The listing builds one solid part. Answer for the finished solid, in the listing's coordinates (mm). A direction names the side the tool comes from. Coordinates: 2 decimals unless noted, no trailing zeros. Write each loop counter-clockwise with the first axis right and the second up, starting at its lowest first coordinate (ties: lowest second). Pieces come first, ordered by that corner, then holes. Notation, with made-up numbers: M 59.25,85 L 112.25,85 A8 cw 112.25,94 Z; hole C 65.5,-29.5 d4. An arc over 180 degrees is marked long. Answer as CSV lines item,"result".
```python
from build123d import *

# Parameters (mm, degrees)
F0_W     = 31.75
F0_H     = 31.75
F1_DEPTH = 1.905
F2_R     = 14.478
F3_DEPTH = 0.889
F5_D     = 1.5875
F6_R     = 1.5875
F7_DEPTH = 3.811
F8_R     = 3.175
F8_R_2   = 1.5875
F9_DEPTH = 2.54


with BuildPart() as f1:
    # F0 (on Front) → F1 (new body, symmetric)
    with BuildSketch(Plane.XZ):
        Rectangle(F0_W, F0_H)
    extrude(amount=F1_DEPTH, both=True)

    # F2 (on face) → F3 (cut)
    with BuildSketch(Plane(origin=(0, 1.905, 0), x_dir=(-1, 0, 0), z_dir=(0, 1, 0))):
        Circle(F2_R)
    extrude(amount=-F3_DEPTH, mode=Mode.SUBTRACT)

    # F5 (through all)
    with Locations(Plane.XZ.offset(1.905)):
        with Locations((-13.335, 13.335), (13.335, 13.335), (13.335, -13.335), (-13.335, -13.335)):
            Hole(F5_D / 2)

    # F6 (on face) → F7 (cut, through all)
    with BuildSketch(Plane.XZ.offset(1.905)):
        Circle(F6_R)
    extrude(amount=-F7_DEPTH, mode=Mode.SUBTRACT)

    # F8 (on face) → F9 (join)
    with BuildSketch(Plane.XZ.offset(1.905)):
        Circle(F8_R)
        Circle(F8_R_2, mode=Mode.SUBTRACT)
    extrude(amount=F9_DEPTH)


solid = f1.part
```
Q1. Find section D-D (x = 6.5). Give the vertices of the cut face in (y, z) (3 decimals), and give its area (3 significant figures).
Output:
outline,"M -1.905,-15.875 L 1.905,-15.875 L 1.905,-12.937 L 1.016,-12.937 L 1.016,12.937 L 1.905,12.937 L 1.905,15.875 L -1.905,15.875 Z"
area,"98.0 mm2"
Q2. Find section B-B (z = 0). Give the vertices of the cut face in (x, y) (1 decimal).
Output:
outline,"M -15.9,-1.9 L -3.2,-1.9 L -3.2,-4.4 L -1.6,-4.4 L -1.6,1 L -14.5,1 L -14.5,1.9 L -15.9,1.9 Z; M 1.6,-4.4 L 3.2,-4.4 L 3.2,-1.9 L 15.9,-1.9 L 15.9,1.9 L 14.5,1.9 L 14.5,1 L 1.6,1 Z"
Q3. Find section A-A (x = 0). Give the vertices of the cut face in (y, z) (1 decimal).
Output:
outline,"M -4.4,-3.2 L -1.9,-3.2 L -1.9,-15.9 L 1.9,-15.9 L 1.9,-14.5 L 1,-14.5 L 1,-1.6 L -4.4,-1.6 Z; M -4.4,1.6 L 1,1.6 L 1,14.5 L 1.9,14.5 L 1.9,15.9 L -1.9,15.9 L -1.9,3.2 L -4.4,3.2 Z"
Q4. Straight lines are drawn through the part: line 1 (Z direction, x = 0, y = 1.45) (3 decimals); line 2 (Z direction, x = 13, y = 1.5) (3 decimals); line 3 (Y direction, x = -12, z = 15) (3 decimals). For each, find the intervals that lie inside material, in ascending order.
Output:
line 1,"-15.875 to -14.478, 14.478 to 15.875"
line 2,"-15.875 to -14.055, -12.615 to -6.373, 6.373 to 12.615, 14.055 to 15.875"
line 3,"-1.905 to 1.905"
Q5. A flat-ended cylindrical pin translates along its axis: pin 1 Ø4 at (x, z) = (10.5, 5.5) entering from -Y (3 decimals). Find the tip coordinate at first contact, or state that the pin passes through.
Output:
pin 1,"y = -1.905"
Q6. For faces 4 (the cylindrical face through (1.885, 1.467, 14.355)), 5 (the cylindrical face through (13.965, 0.027, -13.818)), determine the directions among +Z, -Z, +X, -X, +Y, -Y from which every point of the face is accessible in a straight line to the end or side of a thin tool.
Output:
face 4,"+Y"
face 5,"+Y, -Y"
Q7. The mould has two halves that part along X. Classify faces 1 (the cylindrical face through (-0.69, -3.16, -3.1)), 2 (the flat face through (-5, 1.905, 14)), 3 (the cylindrical face through (13.92, 0.03, 13.87)): pulls with the +X half, pulls with the -X half, needs draft (parallel to the pull), parting line crosses it, or undercut.
Output:
face 1,"parting line crosses it"
face 2,"needs draft"
face 3,"undercut"
Q8. Find section C-C (y = 0). Give the vertices of the cut face in (x, z) (1 decimal).
Output:
outline,"M -15.9,-15.9 L 15.9,-15.9 L 15.9,15.9 L -15.9,15.9 Z; hole C -13.3,-13.3 d1.6; hole C -13.3,13.3 d1.6; hole C 0,0 d3.2; hole C 13.3,-13.3 d1.6; hole C 13.3,13.3 d1.6"
